```python
from build123d import *

# Parameters (mm, degrees)
F0_R     = 1.85
F1_DEPTH = 1.5
F2_R     = 0.5


with BuildPart() as f1:
    # F0 (on Top) → F1 (new body)
    with BuildSketch(Plane.XY):
        with BuildLine():
            Line((9.725, 0), (0, 0))
            Line((0, 0), (0, -14.989273))
            ThreePointArc((0, -14.989273), (2.266295, -15.928004), (3.205026, -18.194299))
            Line((3.205026, -18.194299), (3.205026, -52.04))
            Line((3.205026, -52.04), (6.311514, -57.417158))
            Line((6.311514, -57.417158), (9.485026, -52.079282))
            Line((9.485026, -52.079282), (9.725, -17.13))
            Line((9.725, -17.13), (8.511168, -15.97041))
            ThreePointArc((8.511168, -15.97041), (7.367764, -14.321087), (6.965, -12.35502))
            Line((6.965, -12.35502), (6.965, -10.141257))
            ThreePointArc((6.965, -10.141257), (7.334825, -8.254069), (8.389591, -6.646053))
            Line((8.389591, -6.646053), (9.725, -5.28))
            Line((9.725, -5.28), (9.725, 0))
        make_face()
        with Locations((7.334825, -3.054033)):
            Circle(F0_R, mode=Mode.SUBTRACT)
        with BuildLine():
            Line((0, -14.989273), (0, 0))
            Line((0, 0), (-9.725, 0))
            Line((-9.725, 0), (-9.725, -5.28))
            Line((-9.725, -5.28), (-8.389591, -6.646053))
            ThreePointArc((-8.389591, -6.646053), (-7.334825, -8.254069), (-6.965, -10.141257))
            Line((-6.965, -10.141257), (-6.965, -12.35502))
            ThreePointArc((-6.965, -12.35502), (-7.367764, -14.321087), (-8.511168, -15.97041))
            Line((-8.511168, -15.97041), (-9.725, -17.13))
            Line((-9.725, -17.13), (-9.485026, -52.079282))
            Line((-9.485026, -52.079282), (-6.311514, -57.417158))
            Line((-6.311514, -57.417158), (-3.205026, -52.04))
            Line((-3.205026, -52.04), (-3.205026, -18.194299))
            ThreePointArc((-3.205026, -18.194299), (-2.266295, -15.928004), (0, -14.989273))
        make_face()
        with Locations((-7.334825, -3.054033)):
            Circle(F0_R, mode=Mode.SUBTRACT)
    extrude(amount=F1_DEPTH)

    # F2
    f2_edges = [f1.edges().sort_by_distance(p)[0] for p in [
        (-6.311514, -57.417158, 0.75),
        (6.311514, -57.417158, 0.75),
    ]]
    fillet(f2_edges, radius=F2_R)


solid = f1.part
```
For this review, take the finished solid that the model builds, in its own axes (mm). A direction names the side the tool comes from. Round coordinates to 2 decimals unless told otherwise and drop trailing zeros. Write each loop counter-clockwise with the first axis right and the second up, starting at its lowest first coordinate (ties: lowest second). Pieces come first, ordered by that corner, then holes. Notation, with made-up numbers: (43.5, 54.25) - (47.5, 54.25) arc R21 cw to (47.5, 75.25) - close; hole circle Ø4 at (58.25, -36.5). An arc over 180 degrees is marked (long way). Put each result on its own line as item: value.
Q1. Mouldability with a two-part tool opening along Y and no side actions: class faces 1 (the face through (9.05, -5.97, 0.74)), 2 (the face through (8.1, -54.41, 0.74)), 3 (the face through (7.325, -8.279, 0.74)), 4 (the face through (3.205, -35, 1)) as released by +Y, released by -Y, zero draft, split by the parting line, or undercut.
Solved:
face 1: undercut
face 2: released by -Y
face 3: undercut
face 4: zero draft
Q2. Insertion check: pin 1 Ø0.8 at (y, z) = (-10.5, 0.5) entering from +X; pin 2 Ø0.8 at (y, z) = (-32.5, 0.5) entering from +X; pin 3 Ø0.8 at (y, z) = (-11, 0.5) entering from -X (3 decimals). Each pin has a flat end and moves straight along its axis. Give the tip position at first contact, or say it passes through.
Solved:
pin 1: stops at x = 6.97
pin 2: stops at x = 9.62
pin 3: stops at x = -6.965
Q3. Wall thickness on probe 1 along Y at (x, z) = (-7.75, 1.4); probe 2 along X at (y, z) = (-53, 0.8); probe 3 along X at (y, z) = (-31, 1): over which ranges is each line inside the solid? List them lowest first.
Solved:
probe 1: y = -55 to -15.04, -7.45 to -4.86, -1.25 to 0
probe 2: x = -8.94 to -3.76, 3.76 to 8.94
probe 3: x = -9.63 to -3.21, 3.21 to 9.63
Q4. We need section A-A (y = -40.5). Give the boundary of the cut face in (x, z).
Solved:
outline: (-9.56, 0) - (-3.21, 0) - (-3.21, 1.5) - (-9.56, 1.5) - close; (3.21, 0) - (9.56, 0) - (9.56, 1.5) - (3.21, 1.5) - close
Q5. We need section D-D (x = -5). Give the boundary of the cut face in (y, z), and give its area (3 significant figures).
Solved:
outline: (-55.15, 0) - (0, 0) - (0, 1.5) - (-55.15, 1.5) - close
area: 82.7 mm2
Q6. Machinability: for faces 5 (the face through (-9.11, -16.54, 0.74)), 6 (the face through (-4.564, -54.392, 0.74)), 7 (the face through (7.38, -14.35, 0.74)), which of the approach directions +Z, -Z, +X, -X, +Y, -Y give a long, thin tool a straight path to every point of the face, cutting with its end or side? Answer none if there is none.
Solved:
face 5: +Z, -Z, -X
face 6: +Z, -Z, -Y
face 7: +Z, -Z, +X
Q7. We need section B-B (z = 0.95). Give the boundary of the cut face in (x, y) (3 decimals).
Solved:
outline: (-9.725, -17.13) - (-9.485, -52.079) - (-6.747, -56.684) arc R0.5 ccw to (-5.885, -56.678) - (-3.205, -52.04) - (-3.205, -18.194) arc R3.205 cw to (0, -14.989) arc R3.205 cw to (3.205, -18.194) - (3.205, -52.04) - (5.885, -56.678) arc R0.5 ccw to (6.747, -56.684) - (9.485, -52.079) - (9.725, -17.13) - (8.511, -15.97) arc R5 cw to (6.965, -12.355) - (6.965, -10.141) arc R5 cw to (8.39, -6.646) - (9.725, -5.28) - (9.725, 0) - (-9.725, 0) - (-9.725, -5.28) - (-8.39, -6.646) arc R5 cw to (-6.965, -10.141) - (-6.965, -12.355) arc R5 cw to (-8.511, -15.97) - close; hole circle Ø3.7 at (-7.335, -3.054); hole circle Ø3.7 at (7.335, -3.054)
Q8. We need section C-C (y = -24.5). Give the boundary of the cut face in (x, z).
Solved:
outline: (-9.67, 0) - (-3.21, 0) - (-3.21, 1.5) - (-9.67, 1.5) - close; (3.21, 0) - (9.67, 0) - (9.67, 1.5) - (3.21, 1.5) - close
